Can you work these out from the model? Positions are in its coordinate system, mm. A direction names the side the tool comes from. Give positions to 0.01 mm unless a question says otherwise; leave off trailing zeros. Write each loop counter-clockwise with the first axis right and the second up, starting at its lowest first coordinate (ties: lowest second). Pieces come first, ordered by that corner, then holes.
```python
from build123d import *

# Parameters (mm, degrees)
SKETCH2_W           = 88.9
SKETCH2_H           = 44.45
SKETCH2_R           = 6.35
SKETCH2_R_2         = 3.175
BOSS_EXTRUDE1_DEPTH = 6.35
SKETCH3_R           = 22.225
SKETCH3_W           = 44.45
SKETCH3_H           = 60
BOSS_EXTRUDE2_DEPTH = 6.35
CUT_EXTRUDE1_REACH  = 123.079
SKETCH4_R           = 12.5
SKETCH4_W           = 25
SKETCH4_H           = 60
SKETCH4_W_2         = 18.65
SKETCH4_H_2         = 13.900675703
SKETCH5_W           = 9.725
SKETCH5_H           = 8.324324297
BOSS_EXTRUDE3_DEPTH = 6.35
SKETCH6_W           = 12.9
SKETCH6_H           = 6.769792784
BOSS_EXTRUDE4_DEPTH = 57.15


with BuildPart() as part:
    # Sketch2 → Boss-Extrude1 (new body)
    with BuildSketch(Plane(origin=(0, 0, 0), x_dir=(1, 0, 0), z_dir=(0, 1, 0))):
        with Locations((0, 9.525)):
            Rectangle(SKETCH2_W, SKETCH2_H)
        with Locations(Location((0, 0, 0), (0, 0, 270))):
            Circle(SKETCH2_R, mode=Mode.SUBTRACT)
        with Locations(Location((-31.75, 0, 0), (0, 0, 270))):
            Circle(SKETCH2_R_2, mode=Mode.SUBTRACT)
        with Locations(Location((31.75, 0, 0), (0, 0, 90))):
            Circle(SKETCH2_R_2, mode=Mode.SUBTRACT)
    extrude(amount=BOSS_EXTRUDE1_DEPTH)

    # Sketch3 → Boss-Extrude2 (add)
    with BuildSketch(Plane(origin=(25.4, 0, 0), x_dir=(0, 0, -1), z_dir=(1, 0, 0))):
        with Locations((9.525, 66.35)):
            Circle(SKETCH3_R)
        with Locations((9.525, 36.35)):
            Rectangle(SKETCH3_W, SKETCH3_H)
    boss_extrude2 = extrude(amount=BOSS_EXTRUDE2_DEPTH)

    # Cut-Extrude1: up to this face of the body (flat: up to its plane)
    cut_extrude1_end = Plane(part.part.faces().sort_by_distance((25.4, 45.236582144, -9.525))[0])
    # Sketch4 → Cut-Extrude1 (cut, up to the picked face)
    with BuildSketch(Plane(origin=(31.75, 0, 0), x_dir=(0, 0, -1), z_dir=(1, 0, 0)), mode=Mode.PRIVATE) as cut_extrude1_sk1:
        with Locations((9.525, 66.35)):
            Circle(SKETCH4_R)
    cut_extrude1_tool1 = split(extrude(cut_extrude1_sk1.sketch, amount=-CUT_EXTRUDE1_REACH, mode=Mode.PRIVATE), bisect_by=cut_extrude1_end, keep=Keep.BOTH, mode=Mode.PRIVATE)
    # Sketch4 → Cut-Extrude1 (cut, up to the picked face)
    with BuildSketch(Plane(origin=(31.75, 0, 0), x_dir=(0, 0, -1), z_dir=(1, 0, 0)), mode=Mode.PRIVATE) as cut_extrude1_sk2:
        with Locations((9.525, 36.35)):
            Rectangle(SKETCH4_W, SKETCH4_H)
    cut_extrude1_tool2 = split(extrude(cut_extrude1_sk2.sketch, amount=-CUT_EXTRUDE1_REACH, mode=Mode.PRIVATE), bisect_by=cut_extrude1_end, keep=Keep.BOTH, mode=Mode.PRIVATE)
    # Sketch4 → Cut-Extrude1 (cut, up to the picked face)
    with BuildSketch(Plane(origin=(31.75, 0, 0), x_dir=(0, 0, -1), z_dir=(1, 0, 0)), mode=Mode.PRIVATE) as cut_extrude1_sk3:
        with Locations((9.525, 81.624662148)):
            Rectangle(SKETCH4_W_2, SKETCH4_H_2)
    cut_extrude1_tool3 = split(extrude(cut_extrude1_sk3.sketch, amount=-CUT_EXTRUDE1_REACH, mode=Mode.PRIVATE), bisect_by=cut_extrude1_end, keep=Keep.BOTH, mode=Mode.PRIVATE)
    cut_extrude1_1 = cut_extrude1_tool1.solids().sort_by(Axis((31.75, 66.35, -9.525), (-1, 0, 0)))[0]
    add(cut_extrude1_1, mode=Mode.SUBTRACT)
    cut_extrude1_2 = cut_extrude1_tool2.solids().sort_by(Axis((31.75, 36.35, -9.525), (-1, 0, 0)))[0]
    add(cut_extrude1_2, mode=Mode.SUBTRACT)
    cut_extrude1_3 = cut_extrude1_tool3.solids().sort_by(Axis((31.75, 81.624662, -9.525), (-1, 0, 0)))[0]
    add(cut_extrude1_3, mode=Mode.SUBTRACT)
    cut_extrude1 = cut_extrude1_1 + cut_extrude1_2 + cut_extrude1_3  # Cut-Extrude1 as one shape, for the pattern or mirror that repeats it

    # Sketch5 → Boss-Extrude3 (add)
    with BuildSketch(Plane(origin=(31.75, 0, 0), x_dir=(0, 0, -1), z_dir=(1, 0, 0))):
        Polygon((31.75, 86.524117081), (18.85, 86.524117081), (18.85, 74.674324297), (22.025, 74.674324297), (31.75, 74.674324297), align=None)
        with Locations((26.8875, 70.512162149)):
            Rectangle(SKETCH5_W, SKETCH5_H)
    boss_extrude3 = extrude(amount=-BOSS_EXTRUDE3_DEPTH)

    # Mirror1: Boss-Extrude2, Cut-Extrude1, Boss-Extrude3 across plane
    add(boss_extrude2.mirror(Plane(origin=(0, 0, 0), x_dir=(0, 0, 1), z_dir=(1, 0, 0))))
    add(cut_extrude1.mirror(Plane(origin=(0, 0, 0), x_dir=(0, 0, 1), z_dir=(1, 0, 0))), mode=Mode.SUBTRACT)
    add(boss_extrude3.mirror(Plane(origin=(0, 0, 0), x_dir=(0, 0, 1), z_dir=(1, 0, 0))))

    # Sketch6 → Boss-Extrude4 (add)
    with BuildSketch(Plane(origin=(31.75, 0, 0), x_dir=(0, 0, -1), z_dir=(1, 0, 0))):
        with Locations((25.3, 83.139220689)):
            Rectangle(SKETCH6_W, SKETCH6_H)
    extrude(amount=-BOSS_EXTRUDE4_DEPTH)


solid = part.part
```
1) For faces 5 (the face through (28.619, 70.864, 2.131)), 6 (the face through (25.4, 44, -27)), 7 (the face through (-29, 81, -0.2)), which set-ups out of +Z, -Z, +X, -X, +Y, -Y let a thin tool reach every point of the face, with its end or its side?
Values follow:
face 5: +X, -X
face 6: +Z, -Z
face 7: +X, -X, +Y
2) Suppose I cut it at C-C on x = 0. Write out the boundary of the cut face in (y, z), plus the area to 3 significant figures.
Values follow:
outline: (0, -31.75) - (6.35, -31.75) - (6.35, -6.35) - (0, -6.35) - close; (0, 6.35) - (6.35, 6.35) - (6.35, 12.7) - (0, 12.7) - close; (79.75, -31.75) - (86.52, -31.75) - (86.52, -18.85) - (79.75, -18.85) - close
area: 289 mm2
3) Please list where these lines run through material, in increasing order: L1, parallel to X at y = 4, z = 0 (3 decimals); L2, parallel to X at y = 21.5, z = -27.5; L3, parallel to Z at x = 31.75, y = 2.5 (3 decimals).
Values follow:
L1: x = -44.45 to -34.925, -28.575 to -6.35, 6.35 to 28.575, 34.925 to 44.45
L2: x = -31.75 to -25.4, 25.4 to 31.75
L3: z = -31.75 to -3.175, 3.175 to 12.7
4) Suppose I cut it at A-A on x = -21. Write out the boundary of the cut face in (y, z), plus the area to 3 significant figures.
Values follow:
outline: (0, -31.75) - (6.35, -31.75) - (6.35, 12.7) - (0, 12.7) - close; (79.75, -31.75) - (86.52, -31.75) - (86.52, -18.85) - (79.75, -18.85) - close
area: 370 mm2
5) If we mould it in two halves opening along Y, with no side actions, what happens to faces 1 (the face through (0, 86.524, -25)), 2 (the face through (-28.62, 70.74, -21.23)), 3 (the face through (-1, 0, -10)), 4 (the face through (29, 43, -31.75))? For each: +Y half, -Y half, draft (parallel to the pull), parting line (faces both ways), or undercut.
Values follow:
face 1: +Y half
face 2: undercut
face 3: -Y half
face 4: draft
6) Suppose I cut it at B-B on y = 56. Write out the boundary of the cut face in (x, z) (3 decimals), plus the area to 3 significant figures.
Values follow:
outline: (-31.75, -31.75) - (-25.4, -31.75) - (-25.4, -22.025) - (-31.75, -22.025) - close; (-31.75, 2.975) - (-25.4, 2.975) - (-25.4, 12.7) - (-31.75, 12.7) - close; (25.4, -31.75) - (31.75, -31.75) - (31.75, -22.025) - (25.4, -22.025) - close; (25.4, 2.975) - (31.75, 2.975) - (31.75, 12.7) - (25.4, 12.7) - close
area: 247 mm2
7) For pin 1 Ø14.5 at (x, z) = (0, 0) entering from +Y; pin 2 Ø4 at (y, z) = (27.5, -22.5) entering from +X; pin 3 Ø14 at (y, z) = (54.5, -27.5) entering from -X, each with a flat end and sliding along its axis, tell me the tip position at first contact or that it passes through.
Values follow:
pin 1: stops at y = 6.35
pin 2: stops at x = 31.75
pin 3: stops at x = -31.75
8) Suppose I cut it at D-D on y = 81. Write out the boundary of the cut face in (x, z), plus the area to 3 significant figures.
Values follow:
outline: (-31.75, -31.75) - (31.75, -31.75) - (31.75, -18.85) - (-31.75, -18.85) - close; (-31.75, -0.2) - (-25.4, -0.2) - (-25.4, 7.19) - (-31.75, 7.19) - close; (25.4, -0.2) - (31.75, -0.2) - (31.75, 7.19) - (25.4, 7.19) - close
area: 913 mm2
